Geometry: final body of the model. Coordinates: model frame, mm. Face numbers are marked on the shaded views. Give positions to 0.01 mm unless a question says otherwise; leave off trailing zeros. Order: outer loops, then holes, each group sorted by start corner. A loop starts at its lowest first (then second) coordinate and runs counter-clockwise, first axis right, second up. Notation, with made-up numbers: (15.5, 9) -> (33.5, 9) arc R29 cw to (33.5, 36) -> close; hole circle Ø11 at (-8.5, 70). An arc over 180 degrees is marked (long way). One line per item, written item: value. Start each with the question number.
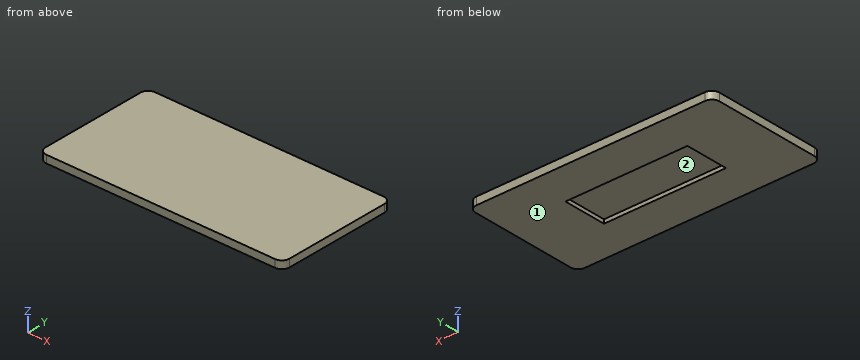
```python
from build123d import *

# Parameters (mm, degrees)
SKETCH_W     = 101.6
SKETCH_H     = 50.8
PAD_DEPTH    = 3.175
FILLET_R     = 3.175
SKETCH001_W  = 50.8
SKETCH001_H  = 18.023603
POCKET_DEPTH = 1.5875


with BuildPart() as part:
    # Sketch → Pad (new body)
    with BuildSketch(Plane.XY):
        Rectangle(SKETCH_W, SKETCH_H)
    extrude(amount=PAD_DEPTH)

    # Fillet
    fillet_edges = [part.edges().sort_by_distance(p)[0] for p in [
        (-50.8, 25.4, 1.5875),
        (50.8, 25.4, 1.5875),
        (50.8, -25.4, 1.5875),
        (-50.8, -25.4, 1.5875),
    ]]
    fillet(fillet_edges, radius=FILLET_R)

    # Sketch001 (on Sketch) → Pocket (cut, symmetric)
    with BuildSketch(Plane(origin=(0, 0, 0), x_dir=(1, 0, 0), z_dir=(0, 0, -1))):
        with Locations((0, 0.329702)):
            Rectangle(SKETCH001_W, SKETCH001_H)
    extrude(amount=POCKET_DEPTH, both=True, mode=Mode.SUBTRACT)


solid = part.part
```
1. Cut plane B-B, the plane y = 5.5. Return loops of the section in (x, z) (1 decimal), then the cut area to 3 significant figures.
2. Draft query along X for the marked faces 1 and 2. Return one class per face: pulls with the +X half, pulls with the -X half, needs draft (parallel to the pull), parting line crosses it, or undercut.
3. Cut plane C-C, the plane x = 16. Return loops of the section in (y, z) (1 decimal), then the cut area to 3 significant figures.
4. Pin query (flat end, axial travel): P1, Ø14.5, axis at x = -4, y = -0.5, coming from the -Z side. Return the tip coordinate at first contact, or that it passes through.
5. Material intervals for L1, parallel to X at y = -22.5, z = 2.2; L2, parallel to Y at x = -24, z = 1.4; L3, parallel to Z at x = -17.5, y = 0 (1 decimal), sorted ascending. Write a range as [from, to].
Answers follow:
1. outline: (-50.8, 0) -> (-25.4, 0) -> (-25.4, 1.6) -> (25.4, 1.6) -> (25.4, 0) -> (50.8, 0) -> (50.8, 3.2) -> (-50.8, 3.2) -> close
1. area: 242 mm²
2. face 1: needs draft
2. face 2: undercut
3. outline: (-25.4, 0) -> (-9.3, 0) -> (-9.3, 1.6) -> (8.7, 1.6) -> (8.7, 0) -> (25.4, 0) -> (25.4, 3.2) -> (-25.4, 3.2) -> close
3. area: 133 mm²
4. P1: stops at z = 1.59
5. L1: x = [-50.79, 50.79]
5. L2: y = [-25.4, -9.34], [8.68, 25.4]
5. L3: z = [1.6, 3.2]
